Could you check a few things on this model? Use its own coordinates, in mm. A direction names the side the tool comes from. Round coordinates to 2 decimals unless told otherwise and drop trailing zeros. Loops run counter-clockwise (first coordinate to the right, second up) from the corner with the lowest first, then second, coordinate; pieces in that order, holes last. Notation, with made-up numbers: (2, 59.5) -> (15, 59.5) arc R8 cw to (15, 70.5) -> close; hole circle Ø3 at (-15, -33.5). An arc over 180 degrees is marked (long way). One line per item, written item: value.
```python
from build123d import *

# Parameters (mm, degrees)
SKETCH2_R                = 5
BOSS_EXTRUDE1_DEPTH      = 10
SKETCH5_R                = 2.4
CUT_EXTRUDE2_DEPTH       = 3
CUT_EXTRUDE5_DEPTH       = 2
CUT_EXTRUDE5_DEPTH_BACK  = 156
BOSS_EXTRUDE2_DEPTH      = 8
BOSS_EXTRUDE2_DEPTH_BACK = 10
SKETCH10_R               = 1.4
CUT_EXTRUDE6_DEPTH       = 8
SKETCH11_R               = 5
BOSS_EXTRUDE3_DEPTH      = 6
SKETCH12_R               = 5
SKETCH12_R_2             = 3
CUT_EXTRUDE8_DEPTH       = 1
SKETCH13_R               = 1.9
CUT_EXTRUDE9_DEPTH       = 5


with BuildPart() as part:
    # Sketch1 → Revolve1 (revolve)
    with BuildSketch(Plane.XY):
        with BuildLine():
            Line((-61.750890187, -47.653200953), (-59.204496779, -47.653200953))
            ThreePointArc((-59.204496779, -47.653200953), (-71.464924193, 25.860483564), (-15, 74.505033387))
            Line((-15, 74.505033387), (-15.394736842, 76.46569216))
            ThreePointArc((-15.394736842, 76.46569216), (-73.070081767, 27.290349038), (-61.750890187, -47.653200953))
        make_face()
    revolve(axis=Axis((0, 0, 0), (0, 1, 0)))

    # Sketch2 → Boss-Extrude1 (add)
    with BuildSketch(Plane.XY.offset(77)):
        Circle(SKETCH2_R)
    extrude(amount=-BOSS_EXTRUDE1_DEPTH)

    # Sketch5 → Cut-Extrude2 (cut)
    with BuildSketch(Plane(origin=(0, 0, 67), x_dir=(-1, 0, 0), z_dir=(0, 0, -1))):
        Circle(SKETCH5_R)
    extrude(amount=-CUT_EXTRUDE2_DEPTH, mode=Mode.SUBTRACT)

    # Sketch8 → Cut-Extrude5 (cut, two sides)
    with BuildSketch(Plane.XY.offset(77)) as cut_extrude5_sk:
        with BuildLine():
            Line((59.204496779, -47.653200953), (-59.204496779, -47.653200953))
            ThreePointArc((-59.204496779, -47.653200953), (0, -9.482803282), (59.204496779, -47.653200953))
        make_face()
    extrude(amount=CUT_EXTRUDE5_DEPTH, mode=Mode.SUBTRACT)
    extrude(cut_extrude5_sk.sketch, amount=-CUT_EXTRUDE5_DEPTH_BACK, mode=Mode.SUBTRACT)

    # Sketch9 → Boss-Extrude2 (add, two sides)
    with BuildSketch(Plane(origin=(0, 0, 0), x_dir=(0, 0, -1), z_dir=(1, 0, 0))) as boss_extrude2_sk:
        Polygon((-24.799638763, 42.367833372), (-18.503698204, 44.659368332), (-18.503698204, 74.505033387), (-27.09103143, 71.379499701), (-35.489739706, 67.690470627), (-39.978084848, 64.869225109), align=None)
    extrude(amount=BOSS_EXTRUDE2_DEPTH)
    extrude(boss_extrude2_sk.sketch, amount=-BOSS_EXTRUDE2_DEPTH_BACK)

    # Sketch10 → Cut-Extrude6 (cut)
    with BuildSketch(Plane(origin=(0, 45.382188608, 16.517765819), x_dir=(1, 0, 0), z_dir=(0, -0.939692621, -0.342020143))):
        with Locations((-4.00206731, 5.513385102)):
            Circle(SKETCH10_R)
        with Locations((2.39793269, 5.513385102)):
            Circle(SKETCH10_R)
    extrude(amount=-CUT_EXTRUDE6_DEPTH, mode=Mode.SUBTRACT)

    # Sketch11 → Boss-Extrude3 (add)
    with BuildSketch(Plane.XY.offset(-77)):
        Circle(SKETCH11_R)
    extrude(amount=BOSS_EXTRUDE3_DEPTH)

    # Sketch12 → Cut-Extrude8 (cut)
    with BuildSketch(Plane.XY.offset(-71)):
        Circle(SKETCH12_R)
        Circle(SKETCH12_R_2, mode=Mode.SUBTRACT)
    extrude(amount=-CUT_EXTRUDE8_DEPTH, mode=Mode.SUBTRACT)

    # Sketch13 → Cut-Extrude9 (cut)
    with BuildSketch(Plane.XY.offset(-71)):
        Circle(SKETCH13_R)
    extrude(amount=-CUT_EXTRUDE9_DEPTH, mode=Mode.SUBTRACT)


solid = part.part
```
(1) On a 3-axis mill with a long thin cutter (end or side, diameter ignored), from which of +Z, -Z, +X, -X, +Y, -Y can I reach the whole of each face in a straight line? I mean faces 1 (the face through (-1.29, 2.024, 68.479)), 2 (the face through (-0.874, 43.498, 21.696)), 3 (the face through (-5.854, -9.747, 76.168)). Say none if no direction works.
Results below:
face 1: none
face 2: -Y
face 3: +Z, -Z, -Y
(2) We'd pull the mould along Y, two halves only. Please class faces 4 (the face through (-1.2, 2.3, 67)), 5 (the face through (0, 0, -76)), 6 (the face through (-5.854, -9.747, -75.807)), 7 (the face through (-1.08, -4.88, -73.94)): +Y half, -Y half, draft (parallel to the pull), parting line (faces both ways), or undercut.
Results below:
face 4: draft
face 5: undercut
face 6: -Y half
face 7: undercut
(3) Imagine slicing it at C-C on z = -29.5. Write out the boundary of the cut face in (x, y).
Results below:
outline: (-57.34, -43.88) arc R65 cw to (-56.19, -41.81) arc R70.04 cw (long way) to (56.19, -41.81) arc R65 cw to (57.34, -43.88) arc R72.21 ccw (long way) to start
(4) Imagine slicing it at B-B on x = 44. Write out the boundary of the cut face in (y, z).
Results below:
outline: (-26.64, -58.64) arc R64.4 ccw (long way) to (-26.64, 58.64) -> (-26.64, 55.95) arc R61.97 cw (long way) to (-26.64, -55.95) -> close
(5) Imagine slicing it at A-A on y = -20. Write out the boundary of the cut face in (x, z).
Results below:
outline: (-35.45, -66.54) -> (-35.45, -64.18) arc R73.32 cw to (-35.45, 64.18) -> (-35.45, 66.54) arc R75.39 ccw to start; (35.45, -66.54) arc R75.39 ccw to (35.45, 66.54) -> (35.45, 64.18) arc R73.32 cw to (35.45, -64.18) -> close
(6) Imagine slicing it at D-D on y = 22. Write out the boundary of the cut face in (x, z), then the cut area to 3 significant figures.
Results below:
outline: circle Ø149.67 at (0, 0); hole circle Ø145.49 at (0, 0)
area: 968 mm²
(7) Please list where these lines run through material, in increasing order: L1, parallel to Y at x = 0, z = 68; L2, parallel to X at y = 51.5, z = 30.5 (3 decimals); L3, parallel to Z at x = 28, y = 57.
Results below:
L1: y = -5 to -2.4, 2.4 to 5, 33.94 to 38.21
L2: x = -50.015 to -46.835, -10 to 8, 46.835 to 50.015
L3: z = -45.29 to -41.75, 41.75 to 45.29
(8) For pin 1 Ø1 at (x, y) = (23, 17) entering from +Z; pin 2 Ø8 at (x, y) = (31, 36.5) entering from -Z; pin 3 Ø6 at (x, z) = (-10, -18) entering from +Y, each with a flat end and sliding along its axis, tell me the tip position at first contact or that it passes through.
Results below:
pin 1: stops at z = 72.76
pin 2: stops at z = -64.48
pin 3: stops at y = 75.99
